from build123d import *

# Parameters (mm, degrees)
SKETCH1_W           = 2.5
SKETCH1_H           = 7
BOSS_EXTRUDE1_DEPTH = 2.5


with BuildPart() as part:
    # Sketch1 → Boss-Extrude1 (new body)
    with BuildSketch(Plane.XY):
        Polygon((-24, 24.4632035), (-24, 21.9632035), (-32, 21.9632035), (-32, 24.4632035), (-42, 24.4632035), (-42, -24.4632035), (42, -24.4632035), (42, 24.4632035), (32, 24.4632035), (32, 21.9632035), (24, 21.9632035), (24, 24.4632035), (16, 24.4632035), (16, 21.9632035), (8, 21.9632035), (8, 24.4632035), (-8, 24.4632035), (-8, 21.9632035), (-16, 21.9632035), (-16, 24.4632035), align=None)
        with Locations((38.75, 4.0367965)):
            Rectangle(SKETCH1_W, SKETCH1_H, mode=Mode.SUBTRACT)
        with Locations((-38.75, -9.9632035)):
            Rectangle(SKETCH1_W, SKETCH1_H, mode=Mode.SUBTRACT)
        with Locations((38.75, -9.9632035)):
            Rectangle(SKETCH1_W, SKETCH1_H, mode=Mode.SUBTRACT)
        with Locations((-38.75, 4.0367965)):
            Rectangle(SKETCH1_W, SKETCH1_H, mode=Mode.SUBTRACT)
    extrude(amount=BOSS_EXTRUDE1_DEPTH)


solid = part.part
The listing builds one solid part. Answer for the finished solid, in the listing's coordinates (mm). A direction names the side the tool comes from. Coordinates: 2 decimals unless noted, no trailing zeros. Loops run counter-clockwise (first coordinate to the right, second up) from the corner with the lowest first, then second, coordinate; pieces in that order, holes last.
1) Find the intervals of material crossed by L1, parallel to X at y = -7.5, z = 0.85; L2, parallel to Y at x = 25, z = 1.4, in increasing order.
2) Find section B-B on x = 31. Write down the section's boundary in (y, z).
3) Find section A-A on z = 1. Give the number of separate pieces and of enclosed holes in the cut face, then the cut area to 3 significant figures.
4) A flat-ended cylindrical pin translates along its axis: pin 1 Ø1.2 at (x, z) = (28.5, 1.5) entering from +Y. Find the tip coordinate at first contact, or state that the pin passes through.
5) A tool of negligible diameter and unlimited length cuts with its end or side. For faces 4 (the face through (-20, 24.463, 1)), 5 (the face through (-39, 0.537, 1)), 6 (the face through (12, 21.963, 1)), from which of +Z, -Z, +X, -X, +Y, -Y can it reach the whole face along a straight path? Write none if from no direction.
6) Determine the mould class of faces 1 (the face through (42, 0, 1)), 2 (the face through (0, 24.463, 1)), 3 (the face through (-16, 23, 1)) for opening direction X: pulls with the +X half, pulls with the -X half, needs draft (parallel to the pull), parting line crosses it, or undercut.
Values:
1. L1: x = -42 to -40, -37.5 to 37.5, 40 to 42
1. L2: y = -24.46 to 21.96
2. outline: (-24.46, 0) - (21.96, 0) - (21.96, 2.5) - (-24.46, 2.5) - close
3. separate pieces: 1
3. enclosed holes: 4
3. area: 3,960 mm2
4. pin 1: stops at y = 21.96
5. face 4: +Z, -Z, +X, -X, +Y
5. face 5: +Z, -Z
5. face 6: +Z, -Z, +Y
6. face 1: pulls with the +X half
6. face 2: needs draft
6. face 3: undercut
